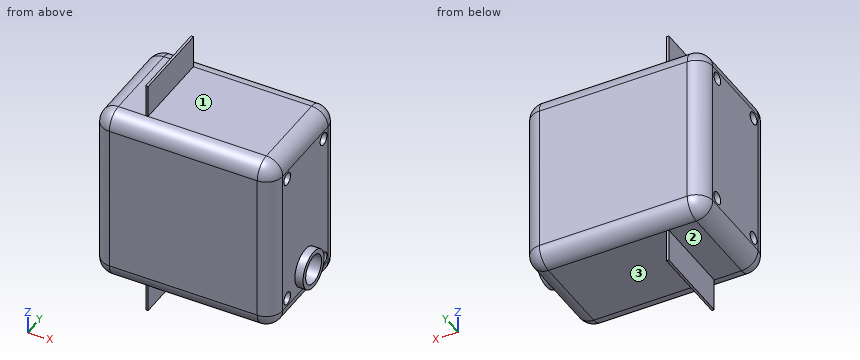
from build123d import *

# Parameters (mm, degrees)
SKETCH1_W                = 22
SKETCH1_H                = 14
BOSS_EXTRUDE1_DEPTH      = 11
FILLET1_R                = 2
SKETCH4_R                = 0.75
CUT_EXTRUDE1_DEPTH       = 28
SKETCH5_R                = 2.324910534
SKETCH5_R_2              = 1.75
BOSS_EXTRUDE2_DEPTH      = 1
CUT_EXTRUDE2_START       = -10
SKETCH5_2_R              = 1.75
CUT_EXTRUDE2_DEPTH       = 10
BOSS_EXTRUDE3_DEPTH      = 4
BOSS_EXTRUDE3_DEPTH_BACK = 26
SKETCH6_W                = 0.286837791
SKETCH6_H                = 10


with BuildPart() as part:
    # Sketch1 → Boss-Extrude1 (new, symmetric)
    with BuildSketch(Plane.XY):
        Rectangle(SKETCH1_W, SKETCH1_H)
    extrude(amount=BOSS_EXTRUDE1_DEPTH, both=True)

    # Fillet1
    fillet1_edges = [part.edges().sort_by_distance(p)[0] for p in [
        (-11, 0, 11),
        (0, -7, 11),
        (11, 0, 11),
        (0, -7, -11),
        (-11, 0, -11),
        (0, 7, -11),
        (11, 0, -11),
        (0, 7, 11),
        (11, -7, 0),
        (-11, -7, 0),
        (-11, 7, 0),
        (11, 7, 0),
    ]]
    fillet(fillet1_edges, radius=FILLET1_R)

    # Sketch4 → Cut-Extrude1 (cut)
    with BuildSketch(Plane(origin=(11, 0, 0), x_dir=(0, 0, -1), z_dir=(1, 0, 0))):
        with Locations((-8, 4)):
            Circle(SKETCH4_R)
        with Locations((-8, -4)):
            Circle(SKETCH4_R)
        with Locations((8, -4)):
            Circle(SKETCH4_R)
        with Locations((8, 4)):
            Circle(SKETCH4_R)
    extrude(amount=-CUT_EXTRUDE1_DEPTH, mode=Mode.SUBTRACT)

    # Sketch5 → Boss-Extrude2 (add)
    with BuildSketch(Plane(origin=(11, 0, 0), x_dir=(0, 0, -1), z_dir=(1, 0, 0))):
        with Locations(Location((6.416436668, 0, 0), (0, 0, 180))):
            Circle(SKETCH5_R)
        with Locations((6.416436668, 0)):
            Circle(SKETCH5_R_2, mode=Mode.SUBTRACT)
    extrude(amount=BOSS_EXTRUDE2_DEPTH)

    # Sketch5<2> → Cut-Extrude2 (cut)
    with BuildSketch(Plane(origin=(11, 0, 0), x_dir=(0, 0, -1), z_dir=(1, 0, 0)).offset(CUT_EXTRUDE2_START)):
        with Locations((6.416436668, 0)):
            Circle(SKETCH5_2_R)
    extrude(amount=CUT_EXTRUDE2_DEPTH, mode=Mode.SUBTRACT)

    # Sketch6 → Boss-Extrude3 (add, two sides: drawn at the far end of the back side and taken through both)
    with BuildSketch(Plane(origin=(0, 0, -11), x_dir=(-1, 0, 0), z_dir=(0, 0, -1)).offset(-BOSS_EXTRUDE3_DEPTH_BACK)):
        with Locations((5.523593607, 0)):
            Rectangle(SKETCH6_W, SKETCH6_H)
    extrude(amount=BOSS_EXTRUDE3_DEPTH + BOSS_EXTRUDE3_DEPTH_BACK)


solid = part.part
Can you work these out from the model? Positions are in its coordinate system, mm. Face numbers are marked on the shaded views. A direction names the side the tool comes from. Round coordinates to 2 decimals unless told otherwise and drop trailing zeros. Write each loop counter-clockwise with the first axis right and the second up, starting at its lowest first coordinate (ties: lowest second). Pieces come first, ordered by that corner, then holes. Notation, with made-up numbers: M -17,16 L 1,16 A37 cw 1,54 Z; hole C 87.25,20 d2. An arc over 180 degrees is marked long. Use CSV: the item, a comma, the result in double quotes.
(1) I'm going to push flat-ended pins straight in: pin 1 (1.2 mm diameter, centred on y = 1.5, z = -12, fed in from -X); pin 2 (2.5 mm diameter, centred on y = -4, z = -8, fed in from +X); pin 3 (4.5 mm diameter, centred on y = -2.5, z = 14, fed in from +X). Where does each tip first touch, or does it pass through?
Check values:
pin 1,"x = -5.67"
pin 2,"x = 11"
pin 3,"x = -5.38"
(2) Imagine slicing it at D-D (z = 8). Write out the boundary of the cut face in (x, y), plus the area to 3 significant figures.
Check values:
outline,"M -11,-5 A2 ccw -9,-7 L 9,-7 A2 ccw 11,-5 L 11,-4.75 L -5.38,-4.75 L -5.38,-3.25 L 11,-3.25 L 11,3.25 L -5.38,3.25 L -5.38,4.75 L 11,4.75 L 11,5 A2 ccw 9,7 L -9,7 A2 ccw -11,5 L -11,4.75 L -5.67,4.75 L -5.67,3.25 L -11,3.25 L -11,-3.25 L -5.67,-3.25 L -5.67,-4.75 L -11,-4.75 Z"
area,"239 mm^2"
(3) On a 3-axis mill with a long thin cutter (end or side, diameter ignored), from which of +Z, -Z, +X, -X, +Y, -Y can I reach the whole of each face in a straight line? I mean the marked faces 1, 2 and 3. Say none if no direction works.
Check values:
face 1,"+Z, +X, +Y, -Y"
face 2,"-Z, -X, +Y, -Y"
face 3,"-Z, +X, +Y, -Y"
(4) Imagine slicing it at C-C (x = -3.75). Write out the boundary of the cut face in (y, z), plus the area to 3 significant figures.
Check values:
outline,"M -7,-9 A2 ccw -5,-11 L 5,-11 A2 ccw 7,-9 L 7,9 A2 ccw 5,11 L -5,11 A2 ccw -7,9 Z; hole C -4,-8 d1.5; hole C -4,8 d1.5; hole C 4,-8 d1.5; hole C 4,8 d1.5"
area,"297 mm^2"
(5) I need wall thicknesses on line 1 along Y through (x, z) = (-7.5, 8); line 2 along Z through (x, y) = (5.25, 4.5); line 3 along Y through (x, z) = (-4.5, 7.5). Which ranges of each line are inside material? Lowest first, please.
Check values:
line 1,"-7 to -4.75, -3.25 to 3.25, 4.75 to 7"
line 2,"-11 to -8.56, -7.44 to 7.44, 8.56 to 11"
line 3,"-7 to -4.56, -3.44 to 3.44, 4.56 to 7"
(6) Imagine slicing it at A-A (x = 7). Write out the boundary of the cut face in (y, z).
Check values:
outline,"M -7,-9 A2 ccw -5,-11 L 5,-11 A2 ccw 7,-9 L 7,9 A2 ccw 5,11 L -5,11 A2 ccw -7,9 Z; hole C -4,-8 d1.5; hole C -4,8 d1.5; hole C 0,-6.42 d3.5; hole C 4,-8 d1.5; hole C 4,8 d1.5"
